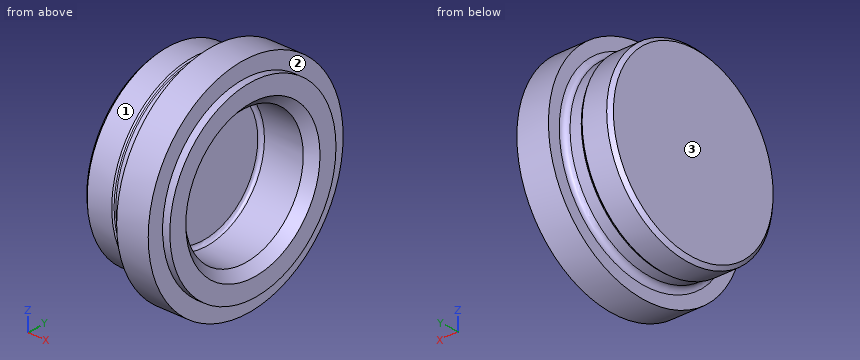
Autodesk Inventor part; units mm, degrees
ref_plane "YZ Plane" through (0, 0, 0) normal (1, 0, 0) x (0, 1, 0)
ref_plane "XZ Plane" through (0, 0, 0) normal (0, 1, 0) x (-1, 0, 0)
ref_plane "XY Plane" through (0, 0, 0) normal (0, 0, 1) x (1, 0, 0)
sketch "Эскиз1" plane through (0, 0, 0) normal (0, 0, 1) x (1, 0, 0)
  line L0 (0, 0) -> (0, 26)
  line L1 (0, 26) -> (8, 26)
  line L2 (8, 26) -> (8.5, 25.5)
  line L3 (8.5, 25.5) -> (13.5, 25.5)
  line L4 (13.5, 25.5) -> (13.5, 30.5)
  line L5 (13.5, 30.5) -> (22.5, 30.5)
  line L6 (22.5, 30.5) -> (22.5, 26)
  line L7 (22.5, 18.5) -> (10, 18.5)
  line L8 (10, 18.5) -> (10, 0)
  line L9 (10, 0) -> (0, 0)
  line L10 (22.5, 26) -> (24.55, 26)
  line L11 (24.55, 26) -> (24.55, 18.5)
  line L12 (24.55, 18.5) -> (22.5, 18.5)
  dimension "d0" = 52
  dimension "d1" = 0.5
  dimension "d2" = 45
  dimension "d3" = 5
  dimension "d4" = 8
  dimension "d5" = 12
  dimension "d6" = 10
  dimension "d7" = 9
  dimension "d8" = 4.5
  dimension "d19" = 22.5
  dimension "d23" = 2.05
revolve "Вращение1" add sketch "Эскиз1" angle 360 about axis through (10, 0, 0) along (-1, 0, 0)
fillet "Сопряжение1" radius 0.5 1 edges at (8.5, -25.5, 0)
fillet "Сопряжение2" radius 1.6 1 edges at (13.5, -25.5, 0)
chamfer "Фаска1" distance 1 angle 45 1 edges at (0, -26, 0)
fillet "Сопряжение3" radius 1 1 edges at (10, -18.5, 0)
chamfer "Фаска4" distance 2.5 angle 45 1 edges at (24.55, -18.5, 0)
equation "\"d5\" = 1.5 * d4"
equation "\"d8\" = 0.5 * d7"
properties part number "Крышка_пром"
The listing builds one solid part. Answer for the finished solid, in the listing's coordinates (mm). Face numbers are marked on the shaded views. A direction names the side the tool comes from. Give positions to 0.01 mm unless a question says otherwise; leave off trailing zeros. Loops run counter-clockwise (first coordinate to the right, second up) from the corner with the lowest first, then second, coordinate; pieces in that order, holes last. Notation, with made-up numbers: (-34, 21.25) - (-13, 21.25) arc R26 ccw to (-13, 50.25) - close; hole circle Ø2 at (-17.75, 43.5). An arc over 180 degrees is marked (long way). Return JSON: item names as keys, results as strings. Group by question number.
1. Find section B-B (x = 3.25). Write down the section's boundary in (y, z), then the cut area to 3 significant figures.
2. Which of the six approach directions +Z, -Z, +X, -X, +Y, -Y give full straight-line access (tool end or side, diameter ignored) to the marked faces 1, 2 and 3?
3. Find section A-A (x = 18). Write down the section's boundary in (y, z), then the cut area to 3 significant figures.
4. Straight lines are drawn through the part: line 1 (Y direction, x = 18.5, z = 0); line 2 (Z direction, x = 15, y = -11.5). For each, find the intervals that lie inside material, in ascending order. Write a range as [from, to].
5. Given pin 1 Ø10.5 at (y, z) = (4, 5.5) entering from +X; pin 2 Ø1.5 at (x, y) = (11, -20.5) entering from -Z; pin 3 Ø12 at (x, y) = (21.5, 0) entering from +Z; pin 4 Ø6 at (y, z) = (6, 22) entering from -X, each flat-ended and moving along its own axis, determine where each tip first touches the part or whether it passes through.
Verdict:
{
 "1": {"outline": "circle Ø52 at (0, 0)", "area": "2,120 mm^2"},
 "2": {"face 1": "-X", "face 2": "+X", "face 3": "+Z, -Z, -X, +Y, -Y"},
 "3": {"outline": "circle Ø61 at (0, 0); hole circle Ø37 at (0, 0)", "area": "1,850 mm^2"},
 "4": {"line 1": "y = [-30.5, -18.5], [18.5, 30.5]", "line 2": "z = [-28.25, -14.49], [14.49, 28.25]"},
 "5": {"pin 1": "stops at x = 10", "pin 2": "stops at z = -16.13", "pin 3": "stops at z = 30.5", "pin 4": "stops at x = 0"}
}
